Input: part model. Units: mm. Frame: model coordinates. A direction names the side the tool comes from. Coordinates: 2 decimals unless noted, no trailing zeros. Order: outer loops, then holes, each group sorted by start corner. A loop starts at its lowest first (then second) coordinate and runs counter-clockwise, first axis right, second up. Notation, with made-up numbers: (83.25, -36.5) -> (96.25, -36.5) arc R19 cw to (96.25, -2.5) -> close; hole circle Ø8 at (18, -12). An arc over 180 degrees is marked (long way). Use one line per item in the form item = value. Start each with the question number.
1) Draft query along Z for faces 1 (the flat face through (-3.153, 2, 15)), 2 (the flat face through (-1, -7, 26)), 3 (the flat face through (-1, -6, 30)), 4 (the cylindrical face through (0.38, -0.73, 22.65)). Return one class per face: pulls with the +Z half, pulls with the -Z half, needs draft (parallel to the pull), parting line crosses it, or undercut.
2) Section query D-D on z = 27.5. Output: boundary loops of the cut face in (x, y).
3) Access query for faces 5 (the flat face through (-1.4, 0.5, 14.8)), 6 (the flat face through (1.647, -1, 18)), 7 (the flat face through (-3, 0, 15)). Directions: +Z, -Z, +X, -X, +Y, -Y. A direction counts if a zero-diameter tool reaches every point of the face in a straight line with its end or side. Return the directions, or none.
4) Section query B-B on y = -0.5. Output: boundary loops of the cut face in (x, z).
5) Ray query, line 1 along X through (y, z) = (-0.15, 8.35); line 2 along X through (y, z) = (-1.4, 11.85); line 3 along Y through (x, z) = (-0.5, 28.5). Return the intervals inside material, ascending.
6) Section query C-C on x = -1.5. Output: boundary loops of the cut face in (y, z), then the cut area to 3 significant figures.
7) Section query A-A on z = 11.85. Output: boundary loops of the cut face in (x, y), then the cut area to 4 significant figures.
8) Pin query (flat end, axial travel): pin 1 (3.5 mm diameter, centred on x = -1, z = 18.5, fed in from -Y); pin 2 (1 mm diameter, centred on x = -1, z = 14, fed in from +Y); pin 3 (4 mm diameter, centred on x = -2, y = -5.5, fed in from -Z). Return the tip coordinate at first contact, or that it passes through.
from build123d import *

# Parameters (mm, degrees)
BOSS_EXTRUDE1_DEPTH   = 30
SKETCH3_R             = 1
CUT_EXTRUDE1_DEPTH    = 10
M2_TAPPED_HOLE1_D     = 1.6
M2_TAPPED_HOLE1_DEPTH = 5.2
M2_TAPPED_HOLE1_TIP   = 0.480688495
SKETCH2_W             = 8
SKETCH2_H             = 4
BOSS_EXTRUDE2_DEPTH   = 10
CHAMFER1_SIZE         = 0.5


with BuildPart() as part:
    # Sketch1 → Boss-Extrude1 (new body)
    with BuildSketch(Plane.XY):
        Polygon((-5.152542373, 3), (-3.152542373, 3), (-3.152542373, 0), (-2.152542373, 0), (-2.152542373, 0.5), (2.847457627, 0.5), (2.847457627, -2), (-5.152542373, -2), align=None)
    extrude(amount=BOSS_EXTRUDE1_DEPTH)

    # Sketch3 → Cut-Extrude1 (cut)
    with BuildSketch(Plane(origin=(0, 0.5, 0), x_dir=(1, 0, 0), z_dir=(0, 1, 0))):
        with Locations((0.347457627, -11.85)):
            Circle(SKETCH3_R)
        with BuildLine():
            Line((-0.952542373, -21.35), (-0.952542373, -15.35))
            ThreePointArc((-0.952542373, -15.35), (0.347457627, -14.05), (1.647457627, -15.35))
            Line((1.647457627, -15.35), (1.647457627, -21.35))
            ThreePointArc((1.647457627, -21.35), (0.347457627, -22.65), (-0.952542373, -21.35))
        make_face()
    extrude(amount=-CUT_EXTRUDE1_DEPTH, mode=Mode.SUBTRACT)

    # M2 Tapped Hole1
    with Locations(Plane(origin=(0, 0.5, 0), x_dir=(1, 0, 0), z_dir=(0, 1, 0))):
        with Locations((0.347457627, -4.35), (0.347457627, -8.35)):
            Hole(M2_TAPPED_HOLE1_D / 2, depth=M2_TAPPED_HOLE1_DEPTH)
            with Locations((0, 0, -(M2_TAPPED_HOLE1_DEPTH + M2_TAPPED_HOLE1_TIP / 2))):  # 118° drill point
                Cone(0, M2_TAPPED_HOLE1_D / 2, M2_TAPPED_HOLE1_TIP, mode=Mode.SUBTRACT)

    # Sketch2 → Boss-Extrude2 (add)
    with BuildSketch(Plane.XZ.offset(2)):
        with Locations((-1.152542373, 28)):
            Rectangle(SKETCH2_W, SKETCH2_H)
    extrude(amount=BOSS_EXTRUDE2_DEPTH)

    # Chamfer1
    chamfer1_edges = [part.edges().sort_by_distance(p)[0] for p in [
        (2.847457627, -2, 13),
        (-5.152542373, -2, 13),
    ]]
    chamfer(chamfer1_edges, length=CHAMFER1_SIZE)


solid = part.part
Answers below:
q1.face_1 = needs draft
q1.face_2 = pulls with the -Z half
q1.face_3 = pulls with the +Z half
q1.face_4 = undercut
q2.outline = (-5.15, -12) -> (2.85, -12) -> (2.85, 0.5) -> (-2.15, 0.5) -> (-2.15, 0) -> (-3.15, 0) -> (-3.15, 3) -> (-5.15, 3) -> close
q3.face_5 = +Z, -Z, +X, +Y
q3.face_6 = +Y, -Y
q3.face_7 = +Z, -Z, +Y
q4.outline = (-5.15, 0) -> (2.85, 0) -> (2.85, 30) -> (-5.15, 30) -> close; hole (-0.95, 15.35) arc R1.3 ccw to (1.65, 15.35) -> (1.65, 21.35) arc R1.3 ccw to (-0.95, 21.35) -> close; hole circle Ø2 at (0.35, 11.85); hole circle Ø1.6 at (0.35, 4.35); hole circle Ø1.6 at (0.35, 8.35)
q5.line_1 = -5.15 to -0.45, 1.15 to 2.85
q5.line_2 = -5.15 to -0.65, 1.35 to 2.85
q5.line_3 = -12 to 0.5
q6.outline = (-12, 26) -> (-2, 26) -> (-2, 0) -> (0.5, 0) -> (0.5, 30) -> (-12, 30) -> close
q6.area = 115 mm^2
q7.outline = (-5.15, -1.5) -> (-4.65, -2) -> (-0.65, -2) -> (-0.65, 0.5) -> (-2.15, 0.5) -> (-2.15, 0) -> (-3.15, 0) -> (-3.15, 3) -> (-5.15, 3) -> close; (1.35, -2) -> (2.35, -2) -> (2.85, -1.5) -> (2.85, 0.5) -> (1.35, 0.5) -> close
q7.area = 19.25 mm^2
q8.pin_1 = -2
q8.pin_2 = 0.5
q8.pin_3 = 26
